Read the model definition and answer for the solid it produces. Units are mm, in the model's axes. Face numbers are marked on the shaded views. A direction names the side the tool comes from. Round coordinates to 2 decimals unless told otherwise and drop trailing zeros. Write each loop counter-clockwise with the first axis right and the second up, starting at its lowest first coordinate (ties: lowest second). Pieces come first, ordered by that corner, then holes.
from build123d import *

# Parameters (mm, degrees)
SKETCH2_R           = 9.25
BOSS_EXTRUDE1_DEPTH = 32.65
FILLET1_R           = 1
SKETCH3_R           = 3.3
CUT_EXTRUDE1_DEPTH  = 0.1
SKETCH4_R           = 3.3
BOSS_EXTRUDE2_DEPTH = 0.5
FILLET2_R           = 0.25


with BuildPart() as part:
    # Sketch2 → Boss-Extrude1 (new body, symmetric)
    with BuildSketch(Plane(origin=(0, 0, 0), x_dir=(1, 0, 0), z_dir=(0, 1, 0))):
        Circle(SKETCH2_R)
    extrude(amount=BOSS_EXTRUDE1_DEPTH, both=True)

    # Fillet1
    fillet1_edges = [part.edges().sort_by_distance(p)[0] for p in [
        (-9.25, -32.65, 0),
        (-9.25, 32.65, 0),
    ]]
    fillet(fillet1_edges, radius=FILLET1_R)

    # Sketch3 → Cut-Extrude1 (cut)
    with BuildSketch(Plane(origin=(0, 32.65, 0), x_dir=(1, 0, 0), z_dir=(0, 1, 0))):
        Circle(SKETCH3_R)
    extrude(amount=-CUT_EXTRUDE1_DEPTH, mode=Mode.SUBTRACT)

    # Sketch4 → Boss-Extrude2 (add)
    with BuildSketch(Plane.XZ.offset(32.65)):
        Circle(SKETCH4_R)
    extrude(amount=BOSS_EXTRUDE2_DEPTH)

    # Fillet2
    fillet2_edges = [part.edges().sort_by_distance(p)[0] for p in [
        (-3.3, -33.15, 0),
    ]]
    fillet(fillet2_edges, radius=FILLET2_R)


solid = part.part
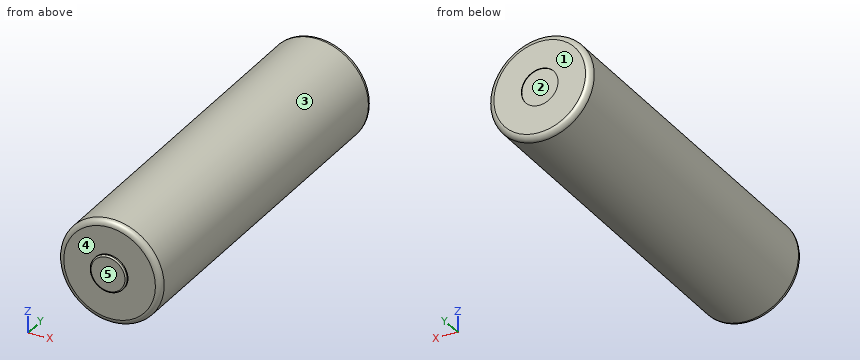
Q1. Section A-A (y = 6) is taken. Determine the outline of the cut face in (x, z).
Verdict:
outline: circle Ø18.5 at (0, 0)
Q2. Flat-ended cylindrical pins translate along their axes: pin 1 Ø4 at (x, y) = (6.5, -9.5) entering from -Z; pin 2 Ø1 at (x, y) = (3.5, 13) entering from +Z; pin 3 Ø5 at (x, y) = (4.5, 10.5) entering from +Z. Find the tip coordinate at first contact, or state that the pin passes through.
Verdict:
pin 1: stops at z = -8.08
pin 2: stops at z = 8.75
pin 3: stops at z = 9.03
Q3. Which of the six approach directions +Z, -Z, +X, -X, +Y, -Y give full straight-line access (tool end or side, diameter ignored) to the marked faces 4 and 5?
Verdict:
face 4: -Y
face 5: +Z, -Z, +X, -X, -Y
Q4. Determine the mould class of the marked faces 1, 2 and 3 for opening direction Z: pulls with the +Z half, pulls with the -Z half, needs draft (parallel to the pull), parting line crosses it, or undercut.
Verdict:
face 1: needs draft
face 2: undercut
face 3: parting line crosses it
Q5. Straight lines are drawn through the part: probe 1 along Y at (x, z) = (-2.75, 7); probe 2 along Y at (x, z) = (2.25, -1); probe 3 along Z at (x, y) = (0.5, 20.5). For each, find the intervals that lie inside material, in ascending order.
Verdict:
probe 1: y = -32.65 to 32.65
probe 2: y = -33.15 to 32.55
probe 3: z = -9.24 to 9.24
